Design review of the part shown in the three views and the two pictorial views. Dimensions are in mm from the part's minimum x, y and z. A direction names the side the tool comes from. Round coordinates to 2 decimals unless told otherwise and drop trailing zeros. Order: outer loops, then holes, each group sorted by start corner. A loop starts at its lowest first (then second) coordinate and runs counter-clockwise, first axis right, second up. Notation, with made-up numbers: (57.25, -21) - (68.25, -21) arc R33 cw to (68.25, 15) - close; hole circle Ø5 at (-18.5, 4.25). An arc over 180 degrees is marked (long way). Use CSV: the item, a comma, the result in double quotes.
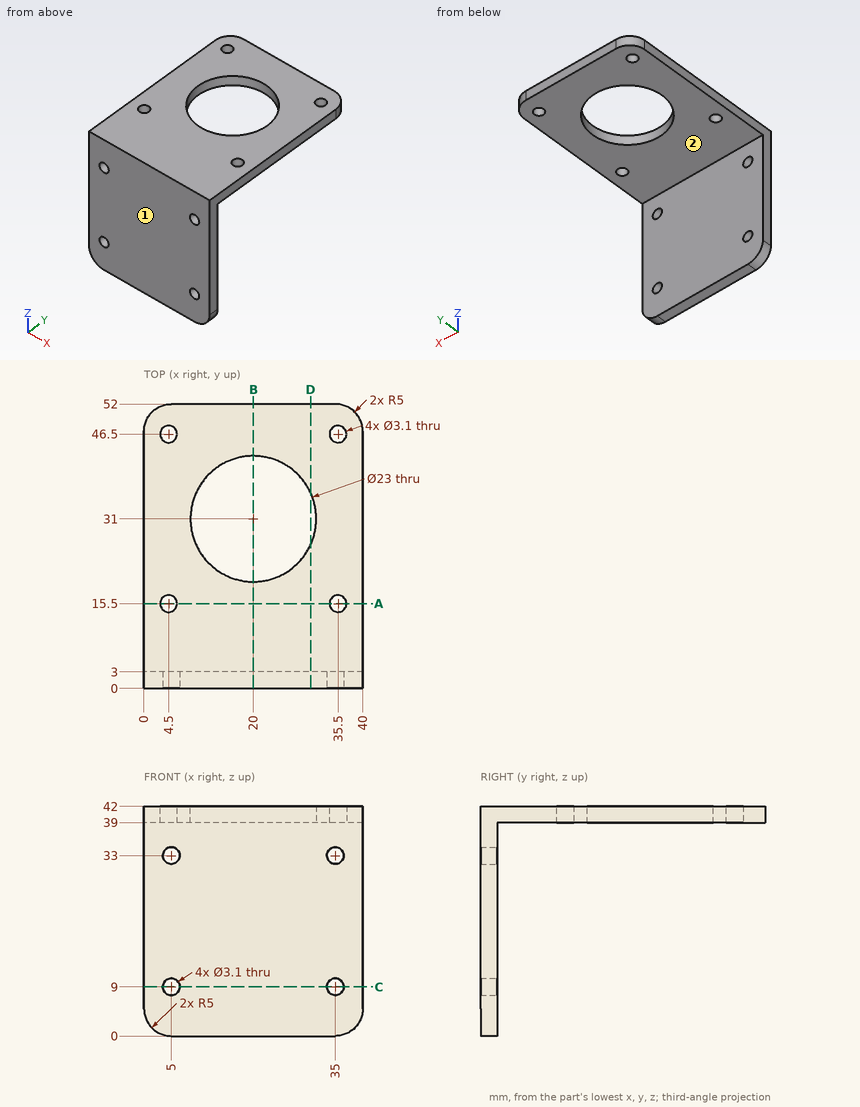
1) To check wall thickness, follow L1, parallel to Z at x = 5, y = 2.35; L2, parallel to X at y = 1, z = 9; L3, parallel to Y at x = 4.5, z = 40.75. State the ranges of each line that lie inside material, in increasing order. Write a range as from..to.
Data:
L1,"z = 0..7.45, 10.55..31.45, 34.55..42"
L2,"x = 0..3.45, 6.55..33.45, 36.55..40"
L3,"y = 0..13.95, 17.05..44.95, 48.05..51.97"
2) We need section D-D (x = 30.5). Give the boundary of the cut face in (y, z), then the cut area to 3 significant figures.
Data:
outline,"(0, 0) - (3, 0) - (3, 39) - (26.31, 39) - (26.31, 42) - (0, 42) - close; (35.69, 39) - (52, 39) - (52, 42) - (35.69, 42) - close"
area,"245 mm2"
3) For the marked faces 1 and 2, list the 3-axis set-ups (+Z, -Z, +X, -X, +Y, -Y) from which the entire face can be reached by the end or side of a thin tool; tool diameter is ignored.
Data:
face 1,"+Z, -Z, +X, -X, -Y"
face 2,"-Z, +X, -X, +Y"
4) We need section C-C (z = 9). Give the boundary of the cut face in (x, y), then the cut area to 3 significant figures.
Data:
outline,"(0, 0) - (3.45, 0) - (3.45, 3) - (0, 3) - close; (6.55, 0) - (33.45, 0) - (33.45, 3) - (6.55, 3) - close; (36.55, 0) - (40, 0) - (40, 3) - (36.55, 3) - close"
area,"101 mm2"
5) Insertion check: pin 1 Ø3.5 at (x, y) = (35.5, 15.5) entering from -Z; pin 2 Ø11.5 at (x, z) = (14.5, 17.5) entering from +Y. Each pin has a flat end and moves straight along its axis. Give the tip position at first contact, or say it passes through.
Data:
pin 1,"stops at z = 39"
pin 2,"stops at y = 3"
6) We need section B-B (x = 20). Give the boundary of the cut face in (y, z).
Data:
outline,"(0, 0) - (3, 0) - (3, 39) - (19.5, 39) - (19.5, 42) - (0, 42) - close; (42.5, 39) - (52, 39) - (52, 42) - (42.5, 42) - close"
7) We need section A-A (y = 15.5). Give the boundary of the cut face in (x, z).
Data:
outline,"(0, 39) - (2.95, 39) - (2.95, 42) - (0, 42) - close; (6.05, 39) - (33.95, 39) - (33.95, 42) - (6.05, 42) - close; (37.05, 39) - (40, 39) - (40, 42) - (37.05, 42) - close"
